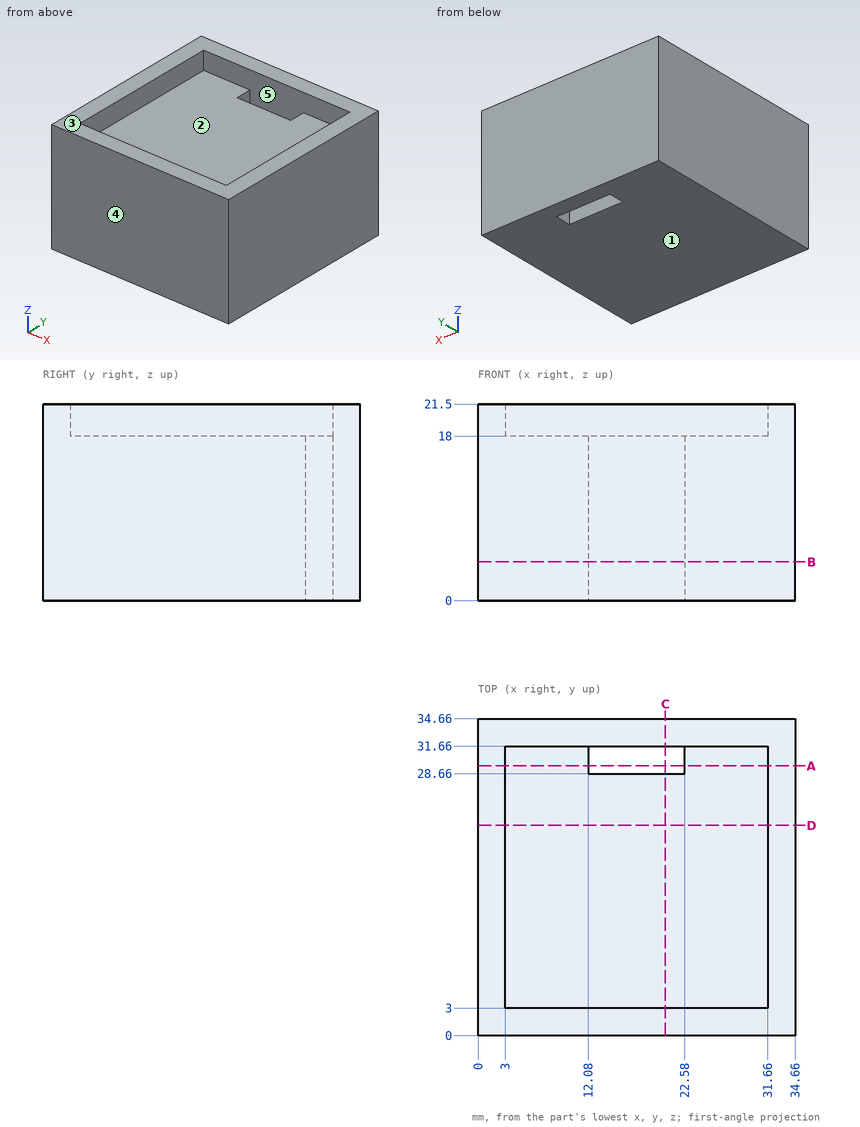
Geometry check sheet. Reference: drawing and pictorial views, mm from the part's lowest x, y, z. A direction names the side the tool comes from. Coordinates: 2 decimals unless noted, no trailing zeros. Write each loop counter-clockwise with the first axis right and the second up, starting at its lowest first coordinate (ties: lowest second). Pieces come first, ordered by that corner, then holes. Notation, with made-up numbers: M 15.5,-10.5 L 56.5,-10.5 A35 cw 56.5,23.5 Z; hole C 70.25,-10 d5. An arc over 180 degrees is marked long. Use one line per item in the form item = value.
Item 1: Sectioned sample at D-D, the plane y = 23. Record the cut outline in (x, z), and give its area (3 significant figures).
Answer below:
outline = M 0,0 L 34.66,0 L 34.66,21.5 L 31.66,21.5 L 31.66,18 L 3,18 L 3,21.5 L 0,21.5 Z
area = 645 mm^2
Item 2: Sectioned sample at A-A, the plane y = 29.5. Record the cut outline in (x, z).
Answer below:
outline = M 0,0 L 12.08,0 L 12.08,18 L 3,18 L 3,21.5 L 0,21.5 Z; M 22.58,0 L 34.66,0 L 34.66,21.5 L 31.66,21.5 L 31.66,18 L 22.58,18 Z
Item 3: Material ranges on L1, parallel to Y at x = 13, z = 11; L2, parallel to Y at x = 14, z = 18.75; L3, parallel to X at y = 31, z = 4.5, recorded low to high. Write a range as from..to.
Answer below:
L1 = 0..28.66, 31.66..34.66
L2 = 0..3, 31.66..34.66
L3 = 0..12.08, 22.58..34.66
Item 4: Sectioned sample at B-B, the plane z = 4.25. Record the cut outline in (x, y).
Answer below:
outline = M 0,0 L 34.66,0 L 34.66,34.66 L 0,34.66 Z; hole M 12.08,28.66 L 22.58,28.66 L 22.58,31.66 L 12.08,31.66 Z
Item 5: Release check for a two-part mould opening along Y. For the marked faces 3, 4 and 5 record: pulls with the +Y half, pulls with the -Y half, needs draft (parallel to the pull), parting line crosses it, or undercut.
Answer below:
face_3 = needs draft
face_4 = pulls with the -Y half
face_5 = undercut
Item 6: Set-up check for the marked faces 1 and 2: record each of +Z, -Z, +X, -X, +Y, -Y from which the full face is reachable in a straight line by a thin tool's end or side.
Answer below:
face_1 = -Z, +X, -X, +Y, -Y
face_2 = +Z
Item 7: Gauge pin test, flat end, axial feed: pin 1 Ø1 at (x, y) = (15, 22) entering from +Z. Record the tip position at first contact, or that the pin passes through.
Answer below:
pin_1 = 18
Item 8: Sectioned sample at C-C, the plane x = 20.5. Record the cut outline in (y, z), and give its area (3 significant figures).
Answer below:
outline = M 0,0 L 28.66,0 L 28.66,18 L 3,18 L 3,21.5 L 0,21.5 Z; M 31.66,0 L 34.66,0 L 34.66,21.5 L 31.66,21.5 Z
area = 591 mm^2
